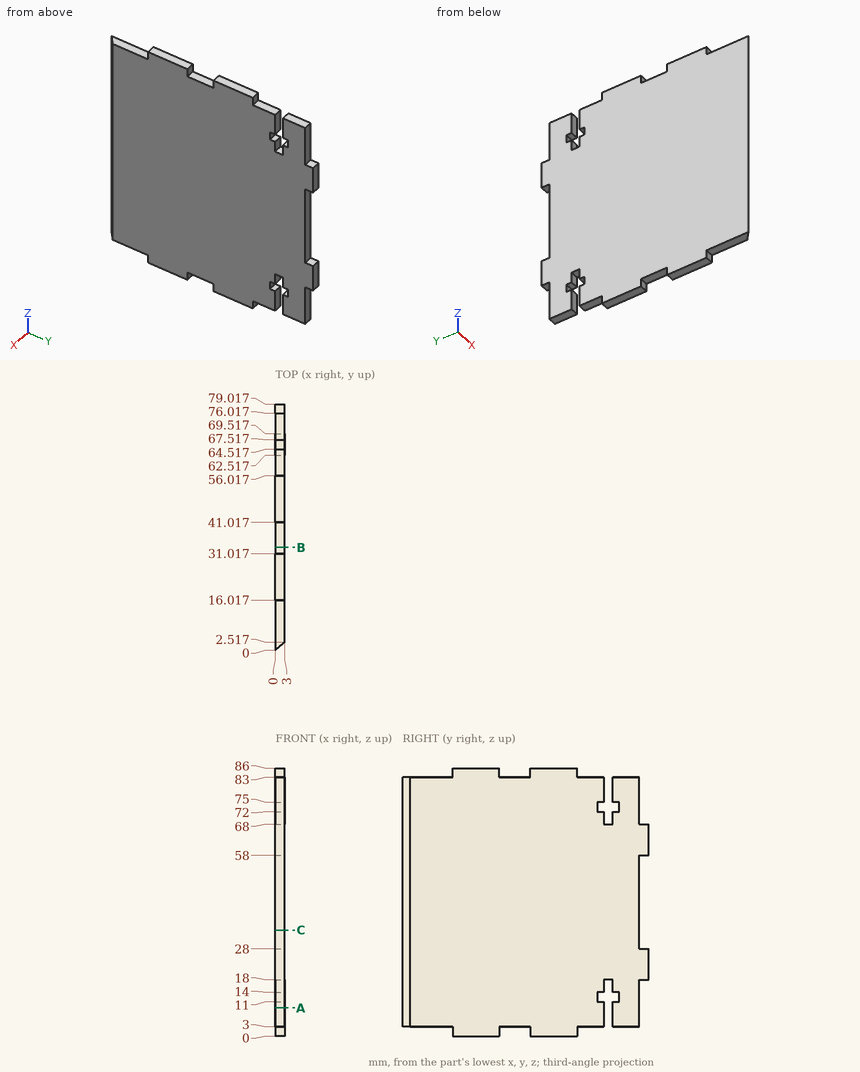
Input: dimensioned drawing with shaded views. Units: mm. Origin: part minimum x, y, z. Round coordinates to 2 decimals unless told otherwise and drop trailing zeros. Order: outer loops, then holes, each group sorted by start corner. A loop starts at its lowest first (then second) coordinate and runs counter-clockwise, first axis right, second up. Notation, with made-up numbers: (-28, -26) - (27, -26) arc R24 ccw to (27, 9) - close; hole circle Ø10 at (85, -36). An arc over 180 degrees is marked (long way). Write item = value, one per line. Start each with the question number.
Q1. Ray query, line 1 (Z direction, x = 2.65, y = 66); line 2 (Z direction, x = 1.6, y = 60); line 3 (Y direction, x = 0.8, z = 15). Return the intervals inside material, ascending. Write a range as from..to.
Q2. Cut plane C-C on z = 34. Return the cut outline in (x, y), and give its area (3 significant figures).
Q3. Cut plane A-A on z = 9. Return the cut outline in (x, y), and give its area (3 significant figures).
Q4. Pin query (flat end, axial travel): pin 1 (1 mm diameter, centred on x = 2, y = 63.5, fed in from +Z); pin 2 (1.5 mm diameter, centred on x = 2, z = 2, fed in from +Y); pin 3 (1.5 mm diameter, centred on x = 2, z = 84.5, fed in from -Y). Return the tip coordinate at first contact, or that it passes through.
Q5. Cut plane B-B on y = 33. Return the cut outline in (x, z).
Outcome:
q1.line_1 = 18..68
q1.line_2 = 3..83
q1.line_3 = 0.67..64.52, 67.52..76.02
q2.outline = (0, 0) - (3, 2.52) - (3, 76.02) - (0, 76.02) - close
q2.area = 224 mm^2
q3.outline = (0, 0) - (3, 2.52) - (3, 64.52) - (0, 64.52) - close; (0, 67.52) - (3, 67.52) - (3, 76.02) - (0, 76.02) - close
q3.area = 215 mm^2
q4.pin_1 = 83
q4.pin_2 = 56.02
q4.pin_3 = 16.02
q5.outline = (0, 3) - (3, 3) - (3, 83) - (0, 83) - close
